Read the model definition and answer for the solid it produces. Units are mm, in the model's axes. A direction names the side the tool comes from. Coordinates: 2 decimals unless noted, no trailing zeros. Loops run counter-clockwise (first coordinate to the right, second up) from the corner with the lowest first, then second, coordinate; pieces in that order, holes last. Notation, with made-up numbers: (25, -27.5) - (77, -27.5) arc R30 ccw to (77, 3.5) - close; hole circle Ø7 at (51, 65). An arc over 180 degrees is marked (long way). Use one line per item in the form item = value.
from build123d import *

# Parameters (mm, degrees)
F0_W     = 10
F0_H     = 10
F1_DEPTH = 5
F3_DEPTH = 5
F2_R     = 2
F4_DEPTH = 25


with BuildPart() as f1:
    # F0 (on Front) → F1 (new body)
    with BuildSketch(Plane.XZ):
        Polygon((-24.7487373415, -31.8198051534), (-5, -40), (-5, -12.0710678119), align=None)
        Polygon((-24.7487373415, 31.8198051534), (-5, 12.0710678119), (-5, 40), align=None)
        Polygon((5, 40), (5, 12.0710678119), (24.7487373415, 31.8198051534), align=None)
        Polygon((-31.8198051534, -38.8908729653), (-24.7487373415, -31.8198051534), (-31.8198051534, -24.7487373415), (-38.8908729653, -31.8198051534), align=None)
        Polygon((24.7487373415, 31.8198051534), (31.8198051534, 24.7487373415), (38.8908729653, 31.8198051534), (31.8198051534, 38.8908729653), align=None)
        Polygon((5, -12.0710678119), (5, -40), (24.7487373415, -31.8198051534), align=None)
        Polygon((31.8198051534, -24.7487373415), (24.7487373415, -31.8198051534), (31.8198051534, -38.8908729653), (38.8908729653, -31.8198051534), align=None)
        Polygon((-40, -5), (-31.8198051534, -24.7487373415), (-12.0710678119, -5), align=None)
        Polygon((-12.0710678119, 5), (-5, 5), (-5, 12.0710678119), (-24.7487373415, 31.8198051534), (-31.8198051534, 24.7487373415), align=None)
        Polygon((-38.8908729653, 31.8198051534), (-31.8198051534, 24.7487373415), (-24.7487373415, 31.8198051534), (-31.8198051534, 38.8908729653), align=None)
        Polygon((-31.8198051534, 24.7487373415), (-40, 5), (-12.0710678119, 5), align=None)
        with Locations((-45, 0)):
            Rectangle(F0_W, F0_H)
        Polygon((-12.0710678119, -5), (-5, -5), (-5, -2.0710678119), (-7.0710678119, 0), align=None)
        with Locations((45, 0)):
            Rectangle(F0_W, F0_H)
        Polygon((5, 2.0710678119), (5, -2.0710678119), (7.0710678119, 0), align=None)
        with Locations((0, 45)):
            Rectangle(F0_W, F0_H)
        Polygon((3.5355339059, -3.5355339059), (5, -2.0710678119), (5, 2.0710678119), (3.5355339059, 3.5355339059), (0, 0), align=None)
        Polygon((-5, -40), (5, -40), (5, -12.0710678119), (0, -7.0710678119), (-5, -12.0710678119), align=None)
        with Locations((0, -45)):
            Rectangle(F0_W, F0_H)
        Polygon((0, -7.0710678119), (5, -12.0710678119), (5, -5), (2.0710678119, -5), align=None)
        Polygon((7.0710678119, 0), (12.0710678119, -5), (40, -5), (40, 5), (12.0710678119, 5), align=None)
        Polygon((5, 5), (5, 2.0710678119), (7.0710678119, 0), (12.0710678119, 5), align=None)
        Polygon((5, -5), (5, -12.0710678119), (24.7487373415, -31.8198051534), (31.8198051534, -24.7487373415), (12.0710678119, -5), align=None)
        Polygon((-2.0710678119, -5), (0, -7.0710678119), (2.0710678119, -5), align=None)
        Polygon((5, 12.0710678119), (5, 5), (12.0710678119, 5), (31.8198051534, 24.7487373415), (24.7487373415, 31.8198051534), align=None)
        Polygon((-40, -5), (-12.0710678119, -5), (-7.0710678119, 0), (-12.0710678119, 5), (-40, 5), align=None)
        Polygon((-5, -5), (-5, -12.0710678119), (0, -7.0710678119), (-2.0710678119, -5), align=None)
        Polygon((5, -2.0710678119), (5, -5), (12.0710678119, -5), (7.0710678119, 0), align=None)
        Polygon((12.0710678119, -5), (31.8198051534, -24.7487373415), (40, -5), align=None)
        Polygon((12.0710678119, 5), (40, 5), (31.8198051534, 24.7487373415), align=None)
        Polygon((-2.0710678119, -5), (2.0710678119, -5), (3.5355339059, -3.5355339059), (0, 0), (-3.5355339059, -3.5355339059), align=None)
        Polygon((0, 7.0710678119), (5, 12.0710678119), (5, 40), (-5, 40), (-5, 12.0710678119), align=None)
        Polygon((-7.0710678119, 0), (-5, -2.0710678119), (-5, 2.0710678119), align=None)
        Polygon((-7.0710678119, 0), (-5, 2.0710678119), (-5, 5), (-12.0710678119, 5), align=None)
        Polygon((-2.0710678119, 5), (2.0710678119, 5), (0, 7.0710678119), align=None)
        Polygon((-5, 2.0710678119), (-5, -2.0710678119), (-3.5355339059, -3.5355339059), (0, 0), (-3.5355339059, 3.5355339059), align=None)
        Polygon((2.0710678119, 5), (5, 5), (5, 12.0710678119), (0, 7.0710678119), align=None)
        Polygon((-5, 12.0710678119), (-5, 5), (-2.0710678119, 5), (0, 7.0710678119), align=None)
        Polygon((-24.7487373415, -31.8198051534), (-5, -12.0710678119), (-5, -5), (-12.0710678119, -5), (-31.8198051534, -24.7487373415), align=None)
        Polygon((-3.5355339059, 3.5355339059), (0, 0), (3.5355339059, 3.5355339059), (2.0710678119, 5), (-2.0710678119, 5), align=None)
        Polygon((-5, 5), (-3.5355339059, 3.5355339059), (-2.0710678119, 5), align=None)
        Polygon((2.0710678119, -5), (5, -5), (3.5355339059, -3.5355339059), align=None)
        Polygon((-5, 5), (-5, 2.0710678119), (-3.5355339059, 3.5355339059), align=None)
        Polygon((3.5355339059, -3.5355339059), (5, -5), (5, -2.0710678119), align=None)
        Polygon((-3.5355339059, -3.5355339059), (-5, -5), (-2.0710678119, -5), align=None)
        Polygon((3.5355339059, 3.5355339059), (5, 2.0710678119), (5, 5), align=None)
        Polygon((3.5355339059, 3.5355339059), (5, 5), (2.0710678119, 5), align=None)
        Polygon((-5, -2.0710678119), (-5, -5), (-3.5355339059, -3.5355339059), align=None)
    extrude(amount=F1_DEPTH)

    # F2 (on face) → F3 (join)
    with BuildSketch(Plane.XZ.offset(5)):
        Polygon((-30.9289321881, -7.0710678119), (0, -38), (7.0710678119, -30.9289321881), (0, -23.8578643763), (-23.8578643763, 0), align=None)
        Polygon((-38, 0), (-30.9289321881, -7.0710678119), (-23.8578643763, 0), (0, 23.8578643763), (-7.0710678119, 30.9289321881), align=None)
        Polygon((0, -23.8578643763), (7.0710678119, -30.9289321881), (38, 0), (30.9289321881, 7.0710678119), (23.8578643763, 0), align=None)
        Polygon((0, 38), (-7.0710678119, 30.9289321881), (0, 23.8578643763), (23.8578643763, 0), (30.9289321881, 7.0710678119), align=None)
    extrude(amount=F3_DEPTH)

    # F2 (on face) → F4 (cut)
    with BuildSketch(Plane.XZ.offset(5)):
        Circle(F2_R)
    extrude(amount=-F4_DEPTH, mode=Mode.SUBTRACT)


solid = f1.part
Item 1: The part is cut by section B-B on x = -35. Give the vertices of the cut face in (y, z), plus the area to 3 significant figures.
Results below:
outline = (-10, -3) - (-5, -3) - (-5, -17.07) - (0, -17.07) - (0, 17.07) - (-5, 17.07) - (-5, 3) - (-10, 3) - close; (-5, -35.71) - (0, -35.71) - (0, -27.93) - (-5, -27.93) - close; (-5, 27.93) - (0, 27.93) - (0, 35.71) - (-5, 35.71) - close
area = 279 mm²
Item 2: Each of these flat-tipped pins is pushed along its axis until it touches: P1, Ø10, axis at x = 34, z = -15.5, coming from the -Y side; P2, Ø5.5, axis at y = -3, z = 44, coming from the -X side; P3, Ø4, axis at x = -10.5, y = -1.5, coming from the +Z side; P4, Ø24, axis at x = -11, z = -11.5, coming from the -Y side. Where does it stop, or does it pass through?
Results below:
P1 = -5
P2 = -5
P3 = 38.55
P4 = -10
Item 3: Find the intervals of material crossed by L1, parallel to Z at x = 0, y = -1.7; L2, parallel to Z at x = 38, y = -4.25; L3, parallel to Z at x = -13, y = -7.5, in increasing order.
Results below:
L1 = -50 to -2, 2 to 50
L2 = -32.71 to -30.93, -9.83 to 9.83, 30.93 to 32.71
L3 = -25 to -10.86, 10.86 to 25
Item 4: Which of the six approach directions +Z, -Z, +X, -X, +Y, -Y give full straight-line access (tool end or side, diameter ignored) to faces 5 (the flat face through (45, -2, 5)), 6 (the flat face through (19, -7, -19)), 7 (the flat face through (18, -5, -22)), 8 (the flat face through (-19, -7, 19)), 9 (the flat face through (-45, -2, -5))?
Results below:
face_5 = +Z, +X, +Y, -Y
face_6 = -Z, +X, -Y
face_7 = -Y
face_8 = +Z, -X, -Y
face_9 = -Z, -X, +Y, -Y
Item 5: The part is cut by section C-C on x = 13. Give the vertices of the cut face in (y, z), plus the area to 3 significant figures.
Results below:
outline = (-10, -25) - (-5, -25) - (-5, -36.69) - (0, -36.69) - (0, 36.69) - (-5, 36.69) - (-5, 25) - (-10, 25) - (-10, 10.86) - (-5, 10.86) - (-5, -10.86) - (-10, -10.86) - close
area = 508 mm²
Item 6: For a pull along X with two mould halves and no side action, classify faces 1 (the flat face through (50, -2, 0)), 2 (the flat face through (-19, -7, -19)), 3 (the flat face through (-28.235, -2.465, 35.306)), 4 (the flat face through (-45, -2, 5)) as +X half, -X half, draft (parallel to the pull), parting line (faces both ways), or undercut.
Results below:
face_1 = +X half
face_2 = -X half
face_3 = undercut
face_4 = draft
Item 7: The part is cut by section D-D on z = -12. Give the vertices of the cut face in (x, y).
Results below:
outline = (-37.1, -5) - (-26, -5) - (-26, -10) - (-11.86, -10) - (-11.86, -5) - (11.86, -5) - (11.86, -10) - (26, -10) - (26, -5) - (37.1, -5) - (37.1, 0) - (-37.1, 0) - close
